Design review of the part built by this model. Coordinates are the model's own, in mm. Face numbers are marked on the shaded views. A direction names the side the tool comes from. Coordinates: 2 decimals unless noted, no trailing zeros. Loops run counter-clockwise (first coordinate to the right, second up) from the corner with the lowest first, then second, coordinate; pieces in that order, holes last. Notation, with made-up numbers: (25.25, 44.25) -> (36.25, 44.25) arc R24 cw to (36.25, 77.25) -> close; hole circle Ø6 at (-20, 67). An arc over 180 degrees is marked (long way). Use CSV: the item, a comma, the result in double quotes.
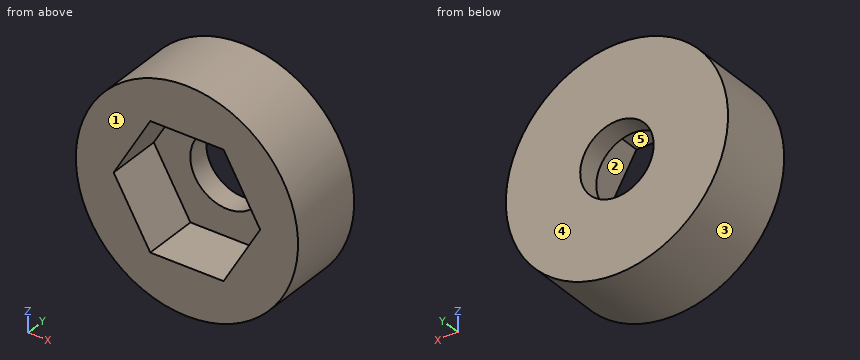
```python
from build123d import *

# Parameters (mm, degrees)
SKETCH_1_R      = 4.990896534
EXTRUDE_1_DEPTH = 2.5
SKETCH_2_R      = 4.990896534
SKETCH_2_R_2    = 1.65
EXTRUDE_2_DEPTH = 1


with BuildPart() as part:
    # 草图1 → 凸台-拉伸1 (new body)
    with BuildSketch(Plane(origin=(0, 0, 0), x_dir=(1, 0, 0), z_dir=(0, 1, 0))):
        with Locations(Location((0, 0, 0), (0, 0, 270))):
            Circle(SKETCH_1_R)
        Polygon((1.645448267, -2.85), (3.290896534, 0), (1.645448267, 2.85), (-1.645448267, 2.85), (-3.290896534, 0), (-1.645448267, -2.85), align=None, mode=Mode.SUBTRACT)
    extrude(amount=EXTRUDE_1_DEPTH)

    # 草图2 → 凸台-拉伸2 (add)
    with BuildSketch(Plane(origin=(0, 2.5, 0), x_dir=(1, 0, 0), z_dir=(0, 1, 0))):
        with Locations(Location((0, 0, 0), (0, 0, 270))):
            Circle(SKETCH_2_R)
        with Locations(Location((0, 0, 0), (0, 0, 270))):
            Circle(SKETCH_2_R_2, mode=Mode.SUBTRACT)
    extrude(amount=EXTRUDE_2_DEPTH)


solid = part.part
```
Item 1: Add section D-D (x = 2.5). Give the boundary of the cut face in (y, z), then the cut area to 3 significant figures.
Checked values:
outline,"(0, -4.32) -> (3.5, -4.32) -> (3.5, 4.32) -> (0, 4.32) -> (0, 1.37) -> (2.5, 1.37) -> (2.5, -1.37) -> (0, -1.37) -> close"
area,"23.4 mm^2"
Item 2: Add section C-C (z = 1.25). Give the boundary of the cut face in (x, y).
Checked values:
outline,"(-4.83, 0) -> (-2.57, 0) -> (-2.57, 2.5) -> (-1.08, 2.5) -> (-1.08, 3.5) -> (-4.83, 3.5) -> close; (1.08, 2.5) -> (2.57, 2.5) -> (2.57, 0) -> (4.83, 0) -> (4.83, 3.5) -> (1.08, 3.5) -> close"
Item 3: Add section A-A (x = 0). Give the boundary of the cut face in (y, z).
Checked values:
outline,"(0, -4.99) -> (3.5, -4.99) -> (3.5, -1.65) -> (2.5, -1.65) -> (2.5, -2.85) -> (0, -2.85) -> close; (0, 2.85) -> (2.5, 2.85) -> (2.5, 1.65) -> (3.5, 1.65) -> (3.5, 4.99) -> (0, 4.99) -> close"
Item 4: Draft analysis for pull direction Z (two halves, no side actions). For the marked faces 3, 4 and 5, state which applies: pulls with the +Z half, pulls with the -Z half, needs draft (parallel to the pull), parting line crosses it, or undercut.
Checked values:
face 3,"parting line crosses it"
face 4,"needs draft"
face 5,"undercut"
Item 5: Clearance check with flat-ended pins moving along their axes: pin 1 (2 mm diameter, centred on y = 0.5, z = -4, fed in from -X); pin 2 (1.5 mm diameter, centred on y = 2, z = -2.5, fed in from +X); pin 3 (1.7 mm diameter, centred on x = 0, z = -1, fed in from -Y); pin 4 (2 mm diameter, centred on x = -0.5, y = 1.5, fed in from -Z). State where each tip first meets the part, or that it passes through.
Checked values:
pin 1,"x = -3.99"
pin 2,"x = 4.67"
pin 3,"y = 2.5"
pin 4,"z = -4.99"
Item 6: To check wall thickness, follow line 1 along X through (y, z) = (3.1, 0); line 2 along Y through (x, z) = (-2.25, -0.5); line 3 along Z through (x, y) = (-0.75, 1.65). State the ranges of each line that lie inside material, in increasing order.
Checked values:
line 1,"-4.99 to -1.65, 1.65 to 4.99"
line 2,"2.5 to 3.5"
line 3,"-4.93 to -2.85, 2.85 to 4.93"
Item 7: Machinability: for the marked faces 1 and 2, which of the approach directions +Z, -Z, +X, -X, +Y, -Y give a long, thin tool a straight path to every point of the face, cutting with its end or side? Answer none if there is none.
Checked values:
face 1,"+Z, -Z, +X, -X, -Y"
face 2,"-Y"
Item 8: Add section B-B (y = 1.25). Give the boundary of the cut face in (x, z).
Checked values:
outline,"circle Ø9.98 at (0, 0); hole (-3.29, 0) -> (-1.65, -2.85) -> (1.65, -2.85) -> (3.29, 0) -> (1.65, 2.85) -> (-1.65, 2.85) -> close"
